from build123d import *

# Parameters (mm, degrees)
F0_R     = 8
F1_DEPTH = 3.5
F2_R     = 8
F3_DEPTH = 1


with BuildPart() as f1:
    # F0 (on Top) → F1 (new body)
    with BuildSketch(Plane.XY):
        with BuildLine():
            ThreePointArc((0, -12.5), (8.838835, -8.838835), (12.5, 0))
            ThreePointArc((12.5, 0), (8.838835, 8.838835), (0, 12.5))
            ThreePointArc((0, 12.5), (-12.5, 0), (0, -12.5))
        make_face()
        Circle(F0_R, mode=Mode.SUBTRACT)
        with BuildLine():
            ThreePointArc((0, -12.5), (-12.5, 0), (0, 12.5))
            Line((0, 12.5), (-35, 12.5))
            Line((-35, 12.5), (-116.388784, 2.506714))
            Line((-116.388784, 2.506714), (-116.388784, -2.506714))
            Line((-116.388784, -2.506714), (-35, -12.5))
            Line((-35, -12.5), (0, -12.5))
        make_face()
    extrude(amount=F1_DEPTH)

    # F2 (on face) → F3 (join)
    with BuildSketch(Plane.XY.offset(3.5)):
        with BuildLine():
            ThreePointArc((0, -12.5), (8.838835, -8.838835), (12.5, 0))
            ThreePointArc((12.5, 0), (8.838835, 8.838835), (0, 12.5))
            ThreePointArc((0, 12.5), (-12.5, 0), (0, -12.5))
        make_face()
        Circle(F2_R, mode=Mode.SUBTRACT)
    extrude(amount=F3_DEPTH)


solid = f1.part
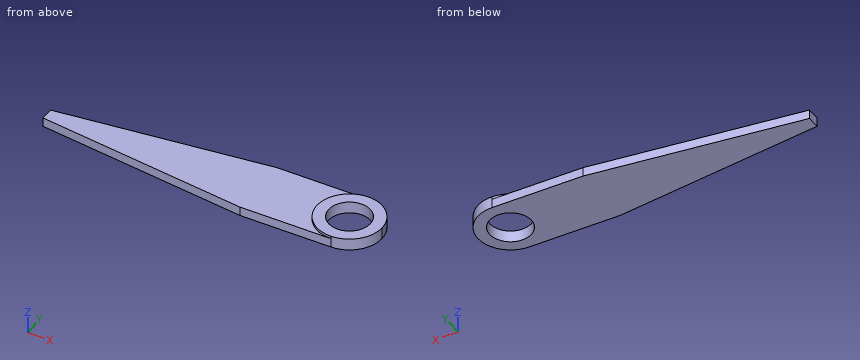
Input: part model. Units: mm. Frame: model coordinates. Coordinates: 2 decimals unless noted, no trailing zeros. Order: outer loops, then holes, each group sorted by start corner. A loop starts at its lowest first (then second) coordinate and runs counter-clockwise, first axis right, second up.
1. Cut plane A-A, the plane z = 1.9. Return loops of the section in (x, y), plus the area to 3 significant figures.
Checked values:
outline: (-116.39, -2.51) - (-35, -12.5) - (0, -12.5) arc R12.5 ccw to (12.5, 0) arc R12.5 ccw to (0, 12.5) - (-35, 12.5) - (-116.39, 2.51) - close; hole circle Ø16 at (0, 0)
area: 2,140 mm2
2. Cut plane B-B, the plane x = -10. Return loops of the section in (y, z), plus the area to 4 significant figures.
Checked values:
outline: (-12.5, 0) - (12.5, 0) - (12.5, 3.5) - (7.5, 3.5) - (7.5, 4.5) - (-7.5, 4.5) - (-7.5, 3.5) - (-12.5, 3.5) - close
area: 102.5 mm2
3. Ray query, line 1 along Y through (x, z) = (0, 1.8); line 2 along Z through (x, y) = (-60, -8); line 3 along X through (y, z) = (-1, 1.1). Return the intervals inside material, ascending.
Checked values:
line 1: y = -12.5 to -8, 8 to 12.5
line 2: z = 0 to 3.5
line 3: x = -116.39 to -7.94, 7.94 to 12.46
4. Contact query for flat-ended pins moving along their axis: P1, Ø2, axis at x = -41.5, z = 1.5, coming from the -Y side; P2, Ø10, axis at x = -103.5, y = 0, coming from the +Z side. Output: stop coordinate, or through.
Checked values:
P1: stops at y = -11.82
P2: stops at z = 3.5
5. Cut plane D-D, the plane x = -53. Return loops of the section in (y, z).
Checked values:
outline: (-10.29, 0) - (10.29, 0) - (10.29, 3.5) - (-10.29, 3.5) - close
6. Cut plane C-C, the plane y = -10.75. Return loops of the section in (x, z).
Checked values:
outline: (-49.25, 0) - (6.38, 0) - (6.38, 4.5) - (-6.38, 4.5) - (-6.38, 3.5) - (-49.25, 3.5) - close
